```python
from build123d import *

# Parameters (mm, degrees)
SKETCH1_W           = 120
SKETCH1_H           = 110
BOSS_EXTRUDE1_DEPTH = 5
SKETCH2_W           = 4
SKETCH2_H           = 110
BOSS_EXTRUDE2_DEPTH = 50
CUT_EXTRUDE1_REACH  = 145.003
SKETCH3_W           = 70.920113649
SKETCH3_H           = 25.988088709


with BuildPart() as part:
    # Sketch1 → Boss-Extrude1 (new body)
    with BuildSketch(Plane(origin=(0, 0, 0), x_dir=(1, 0, 0), z_dir=(0, 1, 0))):
        Rectangle(SKETCH1_W, SKETCH1_H)
    extrude(amount=BOSS_EXTRUDE1_DEPTH)

    # Sketch2 → Boss-Extrude2 (add)
    with BuildSketch(Plane(origin=(0, 5, 0), x_dir=(1, 0, 0), z_dir=(0, 1, 0))):
        with Locations((58, 0)):
            Rectangle(SKETCH2_W, SKETCH2_H)
    extrude(amount=BOSS_EXTRUDE2_DEPTH)

    # Sketch3 → Cut-Extrude1 (cut, up to next)
    with BuildSketch(Plane(origin=(60, 0, 0), x_dir=(0, 0, -1), z_dir=(1, 0, 0)), mode=Mode.PRIVATE) as cut_extrude1_sk1:
        with Locations((9.701412532, 31.435505385)):
            Rectangle(SKETCH3_W, SKETCH3_H)
    cut_extrude1_tool1 = extrude(cut_extrude1_sk1.sketch, amount=-CUT_EXTRUDE1_REACH, mode=Mode.PRIVATE) & part.part
    add(cut_extrude1_tool1.solids().sort_by_distance((60, 31.435505, -9.701413))[0], mode=Mode.SUBTRACT)


solid = part.part
```
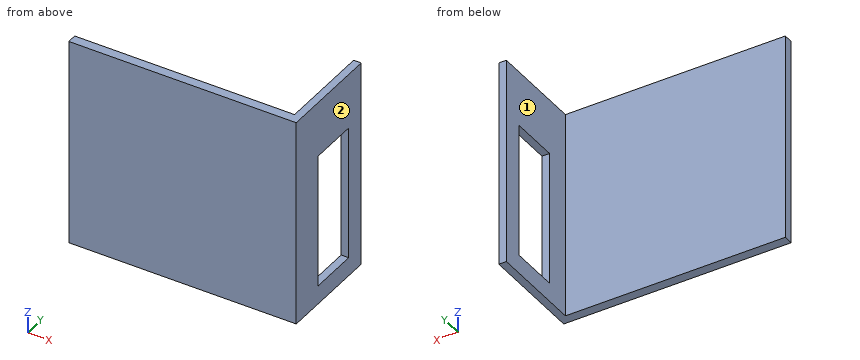
The model under review builds one solid part; all positions refer to its coordinate system, in mm. Face numbers are marked on the shaded views. A direction names the side the tool comes from. Give positions to 0.01 mm unless a question says otherwise; leave off trailing zeros. Loops run counter-clockwise (first coordinate to the right, second up) from the corner with the lowest first, then second, coordinate; pieces in that order, holes last. Notation, with made-up numbers: (86.25, -23) -> (104.25, -23) arc R18 ccw to (104.25, -11) -> close; hole circle Ø5 at (70, 68). An arc over 180 degrees is marked (long way). Use CSV: the item, a comma, the result in double quotes.
1. Consider section B-B, the plane z = -40.5. Write out the cut boundary in (x, y).
Result:
outline,"(-60, 0) -> (60, 0) -> (60, 18.44) -> (56, 18.44) -> (56, 5) -> (-60, 5) -> close; (56, 44.43) -> (60, 44.43) -> (60, 55) -> (56, 55) -> close"
2. Machinability: for the marked faces 1 and 2, which of the approach directions +Z, -Z, +X, -X, +Y, -Y give a long, thin tool a straight path to every point of the face, cutting with its end or side? Answer none if there is none.
Result:
face 1,"+Z, -Z, -X, +Y"
face 2,"+Z, -Z, +X, +Y, -Y"
3. Consider section C-C, the plane z = 38. Write out the cut boundary in (x, y), then the cut area to 3 significant figures.
Result:
outline,"(-60, 0) -> (60, 0) -> (60, 55) -> (56, 55) -> (56, 5) -> (-60, 5) -> close"
area,"800 mm²"
4. To check wall thickness, follow probe 1 along Y at (x, z) = (34, -0.5); probe 2 along X at (y, z) = (44.5, -1). State the ranges of each line that lie inside material, in increasing order. Write a range as from..to.
Result:
probe 1,"y = 0..5"
probe 2,"x = 56..60"
5. Consider section A-A, the plane y = 27. Write out the cut boundary in (x, z).
Result:
outline,"(56, -55) -> (60, -55) -> (60, -45.16) -> (56, -45.16) -> close; (56, 25.76) -> (60, 25.76) -> (60, 55) -> (56, 55) -> close"
6. Consider section D-D, the plane y = 17. Write out the cut boundary in (x, z).
Result:
outline,"(56, -55) -> (60, -55) -> (60, 55) -> (56, 55) -> close"
